```python
from build123d import *

# Parameters (mm, degrees)
RESSALTO_EXTRUS_O1_DEPTH      = 15
RESSALTO_EXTRUS_O1_DEPTH_BACK = 5
ESBO_O1_R                     = 3.571875
ESBO_O1_R_2                   = 3.57
ESBO_O1_R_3                   = 1.25
FILETE1_R                     = 10
CORTE_EXTRUS_O2_START         = -20
CORTE_EXTRUS_O2_DEPTH         = 10
FILETE2_R                     = 10
ESBO_O7_R                     = 0.75
CORTE_EXTRUS_O3_DEPTH         = 259.505319094


with BuildPart() as part:
    # Esboço1 → Ressalto-extrusão1 (new, two sides: drawn at the far end of the back side and taken through both)
    with BuildSketch(Plane(origin=(0, 0, 0), x_dir=(1, 0, 0), z_dir=(0, 1, 0)).offset(-RESSALTO_EXTRUS_O1_DEPTH_BACK)):
        Polygon((210, 50), (105, 75), (0, 75), (0, -75), (105, -75), (210, -50), align=None)
        with Locations(Location((50.8, 0, 0), (0, 0, 270))):
            Circle(ESBO_O1_R, mode=Mode.SUBTRACT)
        with Locations(Location((175.26, 0, 0), (0, 0, 270))):
            Circle(ESBO_O1_R_2, mode=Mode.SUBTRACT)
        with Locations(Location((8.5, -58, 0), (0, 0, 270))):
            Circle(ESBO_O1_R_3, mode=Mode.SUBTRACT)
        with Locations(Location((8.5, -22, 0), (0, 0, 270))):
            Circle(ESBO_O1_R_3, mode=Mode.SUBTRACT)
        with Locations(Location((8.5, 22, 0), (0, 0, 270))):
            Circle(ESBO_O1_R_3, mode=Mode.SUBTRACT)
        with Locations(Location((8.5, 58, 0), (0, 0, 270))):
            Circle(ESBO_O1_R_3, mode=Mode.SUBTRACT)
    extrude(amount=RESSALTO_EXTRUS_O1_DEPTH + RESSALTO_EXTRUS_O1_DEPTH_BACK)

    # Filete1
    filete1_edges = [part.edges().sort_by_distance(p)[0] for p in [
        (0, 5, 75),
        (0, 5, -75),
        (105, 5, -75),
        (210, 5, -50),
        (210, 5, 50),
        (105, 5, 75),
    ]]
    fillet(filete1_edges, radius=FILETE1_R)

    # Esboço6 → Corte-extrusão2 (cut)
    with BuildSketch(Plane(origin=(0, 15, 0), x_dir=(1, 0, 0), z_dir=(0, 1, 0)).offset(CORTE_EXTRUS_O2_START)):
        with BuildLine():
            Line((200, 21.542333602), (200, 42.101412788))
            Line((200, 42.101412788), (103.82593371, 65))
            Line((103.82593371, 65), (65, 65))
            Line((65, 65), (65, 0))
            Line((65, 0), (148.026211544, 0))
            ThreePointArc((148.026211544, 0), (156.322992627, 19.572148207), (176.158102637, 27.218975832))
            Line((176.158102637, 27.218975832), (200, 21.542333602))
        make_face()
        with BuildLine():
            Line((200, -42.101412788), (200, -21.542333602))
            Line((200, -21.542333602), (176.158102637, -27.218975832))
            ThreePointArc((176.158102637, -27.218975832), (156.322992627, -19.572148207), (148.026211544, 0))
            Line((148.026211544, 0), (65, 0))
            Line((65, 0), (65, -65))
            Line((65, -65), (103.82593371, -65))
            Line((103.82593371, -65), (200, -42.101412788))
        make_face()
    extrude(amount=CORTE_EXTRUS_O2_DEPTH, mode=Mode.SUBTRACT)

    # Filete2
    filete2_edges = [part.edges().sort_by_distance(p)[0] for p in [
        (65, 0, 65),
        (65, 0, -65),
        (103.82593371, 0, -65),
        (200, 0, -21.542333602),
        (176.158102637, 0, -27.218975832),
        (200, 0, -42.101412788),
        (200, 0, 42.101412788),
        (176.158102637, 0, 27.218975832),
        (200, 0, 21.542333602),
    ]]
    fillet(filete2_edges, radius=FILETE2_R - 0.0001)  # a hair under: the kernel refuses the full size

    # Esboço7 → Corte-extrusão3 (cut, through all)
    with BuildSketch(Plane(origin=(0, 0, -75), x_dir=(-1, 0, 0), z_dir=(0, 0, -1))):
        with Locations((-40, 5)):
            Circle(ESBO_O7_R)
    extrude(amount=-CORTE_EXTRUS_O3_DEPTH, mode=Mode.SUBTRACT)


solid = part.part
```
The listing builds one solid part. Answer for the finished solid, in the listing's coordinates (mm). A direction names the side the tool comes from. Round coordinates to 2 decimals unless told otherwise and drop trailing zeros. Order: outer loops, then holes, each group sorted by start corner. A loop starts at its lowest first (then second) coordinate and runs counter-clockwise, first axis right, second up. Notation, with made-up numbers: (7, 4.25) - (33, 4.25) arc R13 ccw to (33, 28.25) - close; hole circle Ø5 at (89, -28). An arc over 180 degrees is marked (long way). Put each result on its own line as item: value. Start each with the question number.
(1) Find section B-B (y = 8.25). Give the vertices of the cut face in (x, z).
(2) Given P1, Ø1.5, axis at x = 8.5, z = 58, coming from the +Y side; P2, Ø1, axis at x = 100, z = -55, coming from the -Y side; P3, Ø10, axis at x = 169, y = 12, coming from the -Z side; P4, Ø1.5, axis at x = 168, y = -1, coming from the -Z side, each flat-ended and moving along its own axis, determine where each tip first touches the part or whether it passes through.
(3) For faces 4 (the cylindrical face through (207.79, 5.14, -48.37)), 5 (the flat face through (89, 0, -65)), determine the directions among +Z, -Z, +X, -X, +Y, -Y from which every point of the face is accessible in a straight line to the end or side of a thin tool.
(4) Find section C-C (z = -11). Give the vertices of the cut face in (x, y).
(5) Find section A-A (x = 85.5). Give the vertices of the cut face in (y, z).
(6) Straight lines are drawn through the part: probe 1 along X at (y, z) = (6.75, 0); probe 2 along Z at (x, y) = (188, -2.25); probe 3 along Z at (x, y) = (83.5, 0). For each, find the intervals that lie inside material, in ascending order. Write a range as from..to.
(7) Determine the mould class of faces 1 (the cylindrical face through (54.341, 4.86, -0.465)), 2 (the flat face through (153.56, 4.86, 63.44)), 3 (the flat face through (0, 5, -1)) for opening direction X: released by +X, released by -X, zero draft, split by the parting line, or undercut.
Reply:
1. outline: (0, -65) arc R10 ccw to (10, -75) - (103.83, -75) arc R10 ccw to (106.14, -74.73) - (202.32, -51.83) arc R10 ccw to (210, -42.1) - (210, 42.1) arc R10 ccw to (202.32, 51.83) - (106.14, 74.73) arc R10 ccw to (103.83, 75) - (10, 75) arc R10 ccw to (0, 65) - close; hole circle Ø2.5 at (8.5, -58); hole circle Ø2.5 at (8.5, -22); hole circle Ø2.5 at (8.5, 22); hole circle Ø2.5 at (8.5, 58); hole circle Ø7.14 at (50.8, 0); hole circle Ø7.14 at (175.26, 0)
2. P1: through
2. P2: y = 5
2. P3: z = -60.95
2. P4: z = -60.18
3. face 4: -Z, +X, +Y, -Y
3. face 5: -Y
4. outline: (0, -5) - (65, -5) - (65, 5) - (150.35, 5) - (150.35, -5) - (210, -5) - (210, 15) - (0, 15) - close; hole circle Ø1.5 at (40, 5)
5. outline: (-5, -75) - (15, -75) - (15, 75) - (-5, 75) - (-5, 65) - (5, 65) - (5, -65) - (-5, -65) - close
6. probe 1: 0..47.23, 54.37..171.69, 178.83..210
6. probe 2: -55.24..-44.96, -24.4..24.4, 44.96..55.24
6. probe 3: -75..-65, 65..75
7. face 1: undercut
7. face 2: released by +X
7. face 3: released by -X
